Here's how the part is built. I have some questions about the finished solid (model axes, mm). Round coordinates to 2 decimals unless told otherwise and drop trailing zeros. Write each loop counter-clockwise with the first axis right and the second up, starting at its lowest first coordinate (ties: lowest second). Pieces come first, ordered by that corner, then holes. Notation, with made-up numbers: (40.25, 30.5) - (51.25, 30.5) arc R6 ccw to (51.25, 37.5) - close; hole circle Ø3 at (-11.5, 23.25). An arc over 180 degrees is marked (long way). One line per item, written item: value. Start each with the question number.
Item 1: For P1, Ø8, axis at x = -4.5, y = -39.5, coming from the -Z side, with a flat end and sliding along its axis, tell me the tip position at first contact or that it passes through.
Item 2: Imagine slicing it at B-B, the plane x = -16. Please give me the cut outline in (y, z), then the cut area to 3 significant figures.
Item 3: Imagine slicing it at C-C, the plane y = -142.5. Please give me the cut outline in (x, z), then the cut area to 3 significant figures.
Item 4: Thinking about a two-plate mould opening in Y: for faces 1 (the face through (0, -150, 1)), 2 (the face through (16, -78, 1)), 3 (the face through (0, -74, 0)), which applies, released by +Y, released by -Y, zero draft, split by the parting line, or undercut?
Item 5: If I drill on line 1 (Y direction, x = 16, z = 1.35); line 2 (X direction, y = -50, z = 2.2); line 3 (Y direction, x = 14.5, z = 2.65), over which ranges is the centre line in solid material (lowest first)?
Item 6: Imagine slicing it at A-A, the plane y = -80. Please give me the cut outline in (x, z).
```python
from build123d import *

# Parameters (mm, degrees)
SKETCH1_W           = 50
SKETCH1_H           = 150
BOSS_EXTRUDE1_DEPTH = 3
SKETCH2_R           = 2
CUT_EXTRUDE2_DEPTH  = 4
SKETCH3_R           = 2.1
CUT_EXTRUDE4_DEPTH  = 4


with BuildPart() as part:
    # Sketch1 → Boss-Extrude1 (new body)
    with BuildSketch(Plane.XY):
        with Locations((0, -75)):
            Rectangle(SKETCH1_W, SKETCH1_H)
    extrude(amount=BOSS_EXTRUDE1_DEPTH)

    # Sketch2 → Cut-Extrude2 (cut, through all)
    with BuildSketch(Plane.XY):
        with Locations((-16, -50)):
            Circle(SKETCH2_R)
        with Locations((16, -50)):
            Circle(SKETCH2_R)
        with Locations((-16, -80)):
            Circle(SKETCH2_R)
        with Locations((16, -80)):
            Circle(SKETCH2_R)
    extrude(amount=CUT_EXTRUDE2_DEPTH, mode=Mode.SUBTRACT)

    # Sketch3 → Cut-Extrude4 (cut, through all)
    with BuildSketch(Plane.XY):
        with Locations((-16, -142.5)):
            Circle(SKETCH3_R)
        with Locations((16, -142.5)):
            Circle(SKETCH3_R)
    extrude(amount=CUT_EXTRUDE4_DEPTH, mode=Mode.SUBTRACT)


solid = part.part
```
Values follow:
1. P1: stops at z = 0
2. outline: (-150, 0) - (-144.6, 0) - (-144.6, 3) - (-150, 3) - close; (-140.4, 0) - (-82, 0) - (-82, 3) - (-140.4, 3) - close; (-78, 0) - (-52, 0) - (-52, 3) - (-78, 3) - close; (-48, 0) - (0, 0) - (0, 3) - (-48, 3) - close
2. area: 413 mm^2
3. outline: (-25, 0) - (-18.1, 0) - (-18.1, 3) - (-25, 3) - close; (-13.9, 0) - (13.9, 0) - (13.9, 3) - (-13.9, 3) - close; (18.1, 0) - (25, 0) - (25, 3) - (18.1, 3) - close
3. area: 125 mm^2
4. face 1: released by -Y
4. face 2: undercut
4. face 3: zero draft
5. line 1: y = -150 to -144.6, -140.4 to -82, -78 to -52, -48 to 0
5. line 2: x = -25 to -18, -14 to 14, 18 to 25
5. line 3: y = -150 to -143.97, -141.03 to -81.32, -78.68 to -51.32, -48.68 to 0
6. outline: (-25, 0) - (-18, 0) - (-18, 3) - (-25, 3) - close; (-14, 0) - (14, 0) - (14, 3) - (-14, 3) - close; (18, 0) - (25, 0) - (25, 3) - (18, 3) - close
